Could you check a few things on this model? Use its own coordinates, in mm. Give positions to 0.01 mm unless a question says otherwise; leave off trailing zeros. Order: outer loops, then holes, each group sorted by start corner. A loop starts at its lowest first (then second) coordinate and runs counter-clockwise, first axis right, second up. Notation, with made-up numbers: M -2,-21 L 6,-21 A21 ccw 6,11 Z; hole C 45.5,-28.75 d2. An arc over 180 degrees is marked long. Use a Markdown table: item, result. Add a question column.
Item 1: If we mould it in two halves opening along X, with no side actions, what happens to faces 1 (the face through (0, 5, 70)), 2 (the face through (0, 10, 70)), 3 (the face through (0, 6, 60))? For each: released by +X, released by -X, zero draft, split by the parting line, or undercut.
Item 2: Suppose I cut it at C-C on z = 68.75. Write out the boundary of the cut face in (x, y), plus the area to 3 significant figures.
Item 3: Suppose I cut it at A-A on y = 3. Write out the boundary of the cut face in (x, z).
Item 4: Suppose I cut it at D-D on y = 4.75. Write out the boundary of the cut face in (x, z), plus the area to 3 significant figures.
Item 5: If I drill on L1, parallel to Y at x = 0.25, z = 68.75; L2, parallel to X at y = 2.25, z = 69; L3, parallel to X at y = 2, z = 72.5, over which ranges is the centre line in solid material (lowest first)? Write a range as from..to.
Item 6: I'm going to push flat-ended pins straight in: pin 1 Ø2 at (x, z) = (-3.5, 75) entering from -Y; pin 2 Ø12 at (x, z) = (-7, 67) entering from +Y; pin 3 Ø3 at (x, z) = (-2, 68) entering from +Y. Where does each tip first touch, or does it pass through?
Item 7: Suppose I cut it at B-B on x = 0. Write out the boundary of the cut face in (y, z).
from build123d import *

# Parameters (mm, degrees)
CYLINDER003_R     = 5
CYLINDER003_DEPTH = 20
CYLINDER002_W     = 10
CYLINDER002_H     = 20
CYLINDER002_ANGLE = 180


with BuildPart() as cylinder003:
    # Cylinder003 → Cylinder003 (new body)
    with BuildSketch(Plane.XY):
        Circle(CYLINDER003_R)
    extrude(amount=CYLINDER003_DEPTH)


with BuildPart() as cut:
    # Cylinder002 → Cylinder002 (revolve)
    with BuildSketch(Plane.XZ):
        with Locations((5, 10)):
            Rectangle(CYLINDER002_W, CYLINDER002_H)
    revolve(axis=Axis((0, 0, 0), (0, 0, 1)), revolution_arc=CYLINDER002_ANGLE)

    # Cut: cut Cylinder003
    add(cylinder003.part, mode=Mode.SUBTRACT)


with BuildPart() as cut_1:
    # Cut placement: moved
    add(cut.part.moved(Location((0, 0, 60))))


solid = cut_1.part
Findings below:
| question | item | result |
|---|---|---|
| 1 | face 1 | undercut |
| 1 | face 2 | split by the parting line |
| 1 | face 3 | zero draft |
| 2 | outline | M -10,0 L -5,0 A5 cw 5,0 L 10,0 A10 ccw Z |
| 2 | area | 118 mm^2 |
| 3 | outline | M -9.54,60 L -4,60 L -4,80 L -9.54,80 Z; M 4,60 L 9.54,60 L 9.54,80 L 4,80 Z |
| 4 | outline | M -8.8,60 L -1.56,60 L -1.56,80 L -8.8,80 Z; M 1.56,60 L 8.8,60 L 8.8,80 L 1.56,80 Z |
| 4 | area | 290 mm^2 |
| 5 | L1 | y = 4.99..10 |
| 5 | L2 | x = -9.74..-4.47, 4.47..9.74 |
| 5 | L3 | x = -9.8..-4.58, 4.58..9.8 |
| 6 | pin 1 | stops at y = 2.18 |
| 6 | pin 2 | stops at y = 9.95 |
| 6 | pin 3 | stops at y = 9.99 |
| 7 | outline | M 5,60 L 10,60 L 10,80 L 5,80 Z |
